Check sheet for the modelled part. Datum: model origin and axes. Units: mm. Face numbers are marked on the shaded views. A direction names the side the tool comes from. Give positions to 0.01 mm unless a question says otherwise; leave off trailing zeros. Write each question's results on one line, items separated by ' | '. Start each with the question number.
1. Material ranges on line 1 along Z through (x, y) = (0, 3.5); line 2 along X through (y, z) = (4.5, 1.5); line 3 along X through (y, z) = (4.75, 0.5), recorded low to high.
2. Tool access check on the marked faces 1 and 2. Record the directions out of +Z, -Z, +X, -X, +Y, -Y that give a thin tool (end or side, any length) a straight path to the whole face; none if there is none.
3. Go/stop test with flat-tipped pins: pin 1 (1 mm diameter, centred on x = -2.5, y = 8.5, fed in from +Z); pin 2 (0.5 mm diameter, centred on x = 0, z = 4.5, fed in from -Y); pin 3 (2 mm diameter, centred on x = 2.5, y = 2, fed in from +Z). Record where each tip stops, or that it passes through.
4. Draft check along Z on the marked faces 3, 4, 5 and 6. Enter one of: pulls with the +Z half, pulls with the -Z half, needs draft (parallel to the pull), parting line crosses it, or undercut.
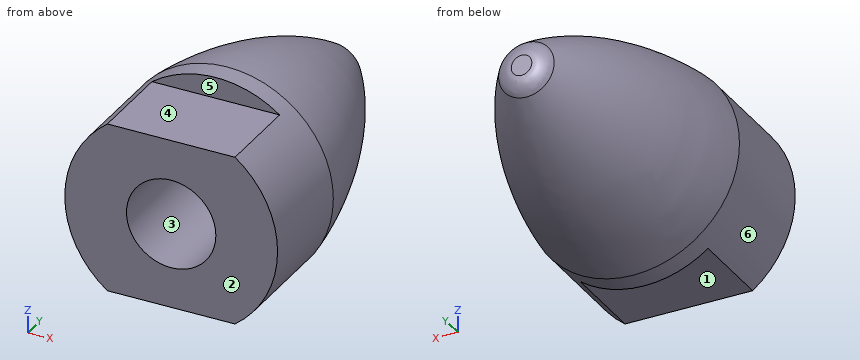
```python
from build123d import *

# Parameters (mm, degrees)
FILLET2_R                 = 1
CUT_EXTRUDE1_DEPTH        = 17.583124103
CUT_EXTRUDE1_DEPTH_BACK   = 17.583124103
SKETCH4_W                 = 3
SKETCH4_H                 = 4
M5X0_8_TAPPED_HOLE1_D     = 4.2
M5X0_8_TAPPED_HOLE1_DEPTH = 8
M5X0_8_TAPPED_HOLE1_TIP   = 1.2618073


with BuildPart() as part:
    # Sketch1 → Revolve2 (revolve)
    with BuildSketch(Plane.XY, mode=Mode.PRIVATE) as revolve2_sk:
        with BuildLine():
            Line((0, 0), (-5, 0))
            Line((-5, 0), (-5, 5))
            ThreePointArc((-5, 5), (-3.621402516, 10.248561006), (-1, 15))
            Line((-1, 15), (0, 15))
            Line((0, 15), (0, 0))
        make_face()
    revolve(revolve2_sk.sketch.rotate(Axis((0, 0, 0), (0, 1, 0)), 270), axis=Axis((0, 0, 0), (0, 1, 0)))

    # Fillet2
    fillet2_edges = [part.edges().sort_by_distance(p)[0] for p in [
        (0, 15, 1),
    ]]
    fillet(fillet2_edges, radius=FILLET2_R)

    # Sketch4 → Cut-Extrude1 (cut, two sides: drawn at the far end of the back side and taken through both)
    with BuildSketch(Plane(origin=(0, 0, 0), x_dir=(0, 0, -1), z_dir=(1, 0, 0)).offset(-CUT_EXTRUDE1_DEPTH_BACK)):
        with Locations((-5.5, 2)):
            Rectangle(SKETCH4_W, SKETCH4_H)
        with Locations((5.5, 2)):
            Rectangle(SKETCH4_W, SKETCH4_H)
    extrude(amount=CUT_EXTRUDE1_DEPTH + CUT_EXTRUDE1_DEPTH_BACK, mode=Mode.SUBTRACT)

    # M5x0.8 Tapped Hole1
    with Locations(Plane(origin=(0, 0, 0), x_dir=(-1, 0, 0), z_dir=(0, -1, 0))):
        with Locations((0, 0)):
            Hole(M5X0_8_TAPPED_HOLE1_D / 2, depth=M5X0_8_TAPPED_HOLE1_DEPTH)
            with Locations((0, 0, -(M5X0_8_TAPPED_HOLE1_DEPTH + M5X0_8_TAPPED_HOLE1_TIP / 2))):  # 118° drill point
                Cone(0, M5X0_8_TAPPED_HOLE1_D / 2, M5X0_8_TAPPED_HOLE1_TIP, mode=Mode.SUBTRACT)


solid = part.part
```
Output values:
1) line 1: -4 to -2.1, 2.1 to 4 | line 2: -4.77 to -1.47, 1.47 to 4.77 | line 3: -4.97 to -2.04, 2.04 to 4.97
2) face 1: -Z, +X, -X, -Y | face 2: +Z, -Z, +X, -X, -Y
3) pin 1: z = 3.78 | pin 2: y = 4 | pin 3: z = 4
4) face 3: undercut | face 4: pulls with the +Z half | face 5: needs draft | face 6: parting line crosses it
